Geometry check sheet. Reference: the model listing, model coordinates, mm. A direction names the side the tool comes from. Round coordinates to 2 decimals unless told otherwise and drop trailing zeros. Order: outer loops, then holes, each group sorted by start corner. A loop starts at its lowest first (then second) coordinate and runs counter-clockwise, first axis right, second up.
Autodesk Fusion 360 part; units mm, degrees
sketch "Sketch1" plane through (0, 0, 0) normal (0, 0, 1) x (1, 0, 0)
  line L0 (46.8447, 156.9249) -> (-67.5, 156.9249)
  line L1 (-67.5, 156.9249) -> (-67.5, 42.5803)
  line L2 (43.8447, 42.5803) -> (43.8447, 156.9249)
  line L3 (-67.5, 42.5803) -> (46.8447, 42.5803)
  circle A0 centre (38.3447, 142.9249) radius 3
  circle A1 centre (38.3447, 113.7526) radius 3
  circle A2 centre (38.3447, 85.7526) radius 3
  circle A3 centre (38.3447, 56.5803) radius 3
  circle A4 centre (-10.3277, 59.7526) radius 2
  circle A5 centre (-64, 46.0803) radius 2
  circle A6 centre (-64, 82.2526) radius 2
  circle A7 centre (-10.3277, 99.7526) radius 2
  circle A8 centre (-10.3277, 139.7526) radius 2
  circle A9 centre (-64, 153.4249) radius 2
  circle A10 centre (-64, 117.2526) radius 2
  dimension "d687" = 6
  dimension "d688" = 4
  dimension "d689" = 10.3277
  dimension "d690" = 54.1723
  dimension "d691" = 53.6723
  dimension "d692" = 48.6723
  dimension "d693" = 114.3447
  dimension "d694" = 57.1723
  dimension "d695" = 17.1723
  dimension "d696" = 97.1723
  dimension "d697" = 57.1723
  dimension "d698" = 59.7526
  dimension "d699" = 93.6723
  dimension "d700" = 83.1723
  dimension "d701" = 80
  dimension "d702" = 57.5
  dimension "d703" = 54
  dimension "d704" = 26
  dimension "d705" = 22.5
  dimension "d706" = 13.6723
  dimension "d707" = 3.1723
extrude "Extrude1" add sketch "Sketch1" along normal blind 2 contours L0 L1 L2 L3 | A4 | A5 | A6 | A7 | A8 | A9 | A10
extrude "Extrude2" add sketch "Sketch1" against normal blind 5 contours A4 | A5 | A6 | A7 | A8 | A9 | A10
(1) Material ranges on line 1 (Y direction, x = -10, z = -1.75); line 2 (Y direction, x = -9.5, z = -1); line 3 (Z direction, x = -57, y = 63.5), recorded low to high.
Returned:
line 1: y = 57.78 to 61.73, 97.78 to 101.73, 137.78 to 141.73
line 2: y = 57.93 to 61.57, 97.93 to 101.57, 137.93 to 141.57
line 3: z = 0 to 2
(2) Sectioned sample at A-A, the plane x = -64. Record the cut outline in (y, z).
Returned:
outline: (42.58, 0) - (44.08, 0) - (44.08, -5) - (48.08, -5) - (48.08, 0) - (80.25, 0) - (80.25, -5) - (84.25, -5) - (84.25, 0) - (115.25, 0) - (115.25, -5) - (119.25, -5) - (119.25, 0) - (151.42, 0) - (151.42, -5) - (155.42, -5) - (155.42, 0) - (156.92, 0) - (156.92, 2) - (42.58, 2) - close
(3) Set-up check for faces 1 (the cylindrical face through (-63.08, 151.65, -2.46)), 2 (the flat face through (-64, 46, -5)): record each of +Z, -Z, +X, -X, +Y, -Y from which the full face is reachable in a straight line by a thin tool's end or side.
Returned:
face 1: -Z
face 2: -Z, +X, -X, +Y, -Y
(4) Draft check along Y on faces 3 (the cylindrical face through (-63.077, 44.306, -2.465)), 4 (the flat face through (-64, 153, -5)). Enter one of: released by +Y, released by -Y, zero draft, split by the parting line, or undercut.
Returned:
face 3: undercut
face 4: zero draft
(5) Sectioned sample at C-C, the plane x = -16. Record the cut outline in (y, z).
Returned:
outline: (42.58, 0) - (156.92, 0) - (156.92, 2) - (42.58, 2) - close
(6) Sectioned sample at B-B, the plane z = -2. Record the cut outline in (x, y), and give its area (3 significant figures).
Returned:
outline: circle Ø4 at (-64, 46.08); circle Ø4 at (-64, 82.25); circle Ø4 at (-64, 117.25); circle Ø4 at (-64, 153.42); circle Ø4 at (-10.33, 59.75); circle Ø4 at (-10.33, 99.75); circle Ø4 at (-10.33, 139.75)
area: 88.0 mm2
(7) Depth check by flat-ended pin: P1, Ø5, axis at x = 38.34, y = 56.58, coming from the +Z side; P2, Ø1, axis at x = 25, y = 94, coming from the -Z side. Enter the tip coordinate at first touch or a pass-through.
Returned:
P1: passes through
P2: stops at z = 0
